```python
from build123d import *

# Parameters (mm, degrees)
SKETCH_1_R          = 1
EXTRUDE_1_DEPTH     = 2
FILLET_1_R          = 3
CUT_EXTRUDE_1_DEPTH = 10
OTHER_1_DEPTH       = 2


# Read off the part's stored shape, not the designer's step: 填充阵列1
with BuildPart() as part:
    # 草图1 → 凸台-拉伸1 (new body)
    with BuildSketch(Plane.XY):
        Polygon((-41.460043107, 0.647951852), (-72.584789341, 2.123935292), (-72.584789341, 63.876064708), (-41.460043107, 65.352048148), align=None)
        with Locations((-67.448676919, 57.358573192)):
            Circle(SKETCH_1_R, mode=Mode.SUBTRACT)
        with Locations((-47.471291497, 58.309400037)):
            Circle(SKETCH_1_R, mode=Mode.SUBTRACT)
        with Locations((-67.448676919, 8.641426808)):
            Circle(SKETCH_1_R, mode=Mode.SUBTRACT)
        with Locations((-47.471291497, 7.690599963)):
            Circle(SKETCH_1_R, mode=Mode.SUBTRACT)
    extrude(amount=EXTRUDE_1_DEPTH)

    # 圆角1
    fillet_1_edges = [part.edges().sort_by_distance(p)[0] for p in [
        (-41.460043107, 0.647951852, 1),
        (-72.584789341, 2.123935292, 1),
        (-72.584789341, 63.876064708, 1),
        (-41.460043107, 65.352048148, 1),
    ]]
    fillet(fillet_1_edges, radius=FILLET_1_R)

    # 草图4 → 切除-拉伸1 (cut)
    with BuildSketch(Plane.XY.offset(2)):
        Polygon((-59.022416224, 33), (-55.022416224, 33), (-55.022416224, 34.154700538), (-57.022416224, 35.309401077), (-59.022416224, 34.154700538), align=None)
        Polygon((-55.022416224, 31.845299462), (-55.022416224, 33), (-59.022416224, 33), (-59.022416224, 31.845299462), (-57.022416224, 30.690598923), align=None)
    extrude(amount=-CUT_EXTRUDE_1_DEPTH, mode=Mode.SUBTRACT)

    # 填充阵列1 outline → 填充阵列1 (cut)
    with BuildSketch(Plane.XY):
        Polygon((-61.084594051, 30.654700538), (-63.084594051, 31.809401077), (-65.084594051, 30.654700538), (-65.084594051, 28.345299462), (-63.084594051, 27.190598923), (-61.084594051, 28.345299462), align=None)
        Polygon((-48.960238398, 37.654700538), (-50.960238398, 38.809401077), (-52.960238398, 37.654700538), (-52.960238398, 35.345299462), (-50.960238398, 34.190598923), (-48.960238398, 35.345299462), align=None)
        Polygon((-48.960238398, 28.345299462), (-48.960238398, 30.654700538), (-50.960238398, 31.809401077), (-52.960238398, 30.654700538), (-52.960238398, 28.345299462), (-50.960238398, 27.190598923), align=None)
        Polygon((-61.084594051, 35.345299462), (-61.084594051, 37.654700538), (-63.084594051, 38.809401077), (-65.084594051, 37.654700538), (-65.084594051, 35.345299462), (-63.084594051, 34.190598923), align=None)
        Polygon((-57.022416224, 51.690598923), (-55.022416224, 52.845299462), (-55.022416224, 55.154700538), (-57.022416224, 56.309401077), (-59.022416224, 55.154700538), (-59.022416224, 52.845299462), align=None)
        Polygon((-57.022416224, 9.690598923), (-55.022416224, 10.845299462), (-55.022416224, 13.154700538), (-57.022416224, 14.309401077), (-59.022416224, 13.154700538), (-59.022416224, 10.845299462), align=None)
        Polygon((-57.022416224, 23.690598923), (-55.022416224, 24.845299462), (-55.022416224, 27.154700538), (-57.022416224, 28.309401077), (-59.022416224, 27.154700538), (-59.022416224, 24.845299462), align=None)
        Polygon((-57.022416224, 16.690598923), (-55.022416224, 17.845299462), (-55.022416224, 20.154700538), (-57.022416224, 21.309401077), (-59.022416224, 20.154700538), (-59.022416224, 17.845299462), align=None)
        Polygon((-57.022416224, 44.690598923), (-55.022416224, 45.845299462), (-55.022416224, 48.154700538), (-57.022416224, 49.309401077), (-59.022416224, 48.154700538), (-59.022416224, 45.845299462), align=None)
        Polygon((-57.022416224, 37.690598923), (-55.022416224, 38.845299462), (-55.022416224, 41.154700538), (-57.022416224, 42.309401077), (-59.022416224, 41.154700538), (-59.022416224, 38.845299462), align=None)
        Polygon((-61.084594051, 51.654700538), (-63.084594051, 52.809401077), (-65.084594051, 51.654700538), (-65.084594051, 49.345299462), (-63.084594051, 48.190598923), (-61.084594051, 49.345299462), align=None)
        Polygon((-48.960238398, 49.345299462), (-48.960238398, 51.654700538), (-50.960238398, 52.809401077), (-52.960238398, 51.654700538), (-52.960238398, 49.345299462), (-50.960238398, 48.190598923), align=None)
        Polygon((-48.960238398, 16.654700538), (-50.960238398, 17.809401077), (-52.960238398, 16.654700538), (-52.960238398, 14.345299462), (-50.960238398, 13.190598923), (-48.960238398, 14.345299462), align=None)
        Polygon((-61.084594051, 14.345299462), (-61.084594051, 16.654700538), (-63.084594051, 17.809401077), (-65.084594051, 16.654700538), (-65.084594051, 14.345299462), (-63.084594051, 13.190598923), align=None)
        Polygon((-48.960238398, 23.654700538), (-50.960238398, 24.809401077), (-52.960238398, 23.654700538), (-52.960238398, 21.345299462), (-50.960238398, 20.190598923), (-48.960238398, 21.345299462), align=None)
        Polygon((-50.960238398, 41.190598923), (-48.960238398, 42.345299462), (-48.960238398, 44.654700538), (-50.960238398, 45.809401077), (-52.960238398, 44.654700538), (-52.960238398, 42.345299462), align=None)
        Polygon((-61.084594051, 23.654700538), (-63.084594051, 24.809401077), (-65.084594051, 23.654700538), (-65.084594051, 21.345299462), (-63.084594051, 20.190598923), (-61.084594051, 21.345299462), align=None)
        Polygon((-63.084594051, 41.190598923), (-61.084594051, 42.345299462), (-61.084594051, 44.654700538), (-63.084594051, 45.809401077), (-65.084594051, 44.654700538), (-65.084594051, 42.345299462), align=None)
    extrude(amount=OTHER_1_DEPTH, mode=Mode.SUBTRACT)


solid = part.part
```
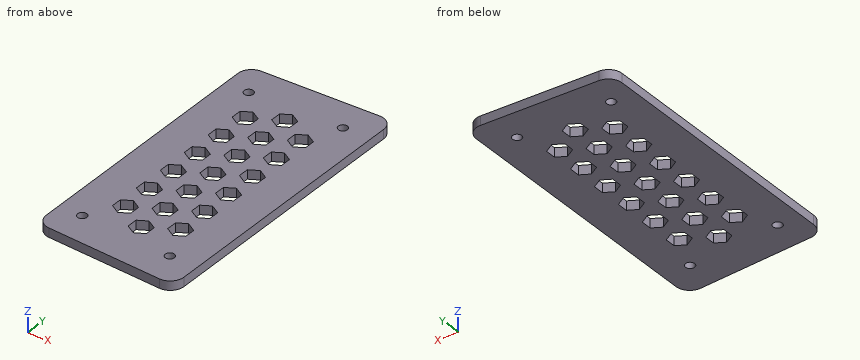
Work out the finished part from the listing and answer in its coordinate system (mm). Give positions to 0.01 mm unless a question says otherwise; leave off trailing zeros. Loops run counter-clockwise (first coordinate to the right, second up) from the corner with the lowest first, then second, coordinate; pieces in that order, holes last. Notation, with made-up numbers: M 85.5,58 L 119.5,58 A23 ccw 119.5,93 Z; hole C 3,38 d10. An arc over 180 degrees is marked long. One line per item, written item: value. Start each with the question number.
1. Find section B-B (z = 0.45). State how many separate pieces and enclosed holes the cut face has, and give its area (3 significant figures).
2. Find section A-A (y = 40). Give the vertices of the cut face in (x, z).
3. Find the intervals of material crossed by probe 1 along X at (y, z) = (36.5, 0.45); probe 2 along X at (y, z) = (17, 0.9); probe 3 along X at (y, z) = (46, 0.5), in increasing order.
Reported:
1. separate pieces: 1
1. enclosed holes: 23
1. area: 1,680 mm²
2. outline: M -72.58,0 L -59.02,0 L -59.02,2 L -72.58,2 Z; M -55.02,0 L -41.46,0 L -41.46,2 L -55.02,2 Z
3. probe 1: x = -72.58 to -65.08, -61.08 to -52.96, -48.96 to -41.46
3. probe 2: x = -72.58 to -64.49, -61.68 to -57.56, -56.49 to -52.36, -49.56 to -41.46
3. probe 3: x = -72.58 to -59.02, -55.02 to -41.46
